```python
from build123d import *

# Parameters (mm, degrees)
F0_R     = 35
F1_DEPTH = 10


with BuildPart() as f1:
    # F0 (on Top) → F1 (new body)
    with BuildSketch(Plane.XY):
        Circle(F0_R)
    extrude(amount=F1_DEPTH)

    # F2 (on Front) → F3 (revolve)
    with BuildSketch(Plane.XZ):
        with BuildLine():
            Line((-26.283575, 70.897411), (-38.094532, 70.897411))
            Line((-38.094532, 70.897411), (-38.094532, 64.87011))
            Line((-38.094532, 64.87011), (-32.239489, 64.87011))
            Line((-32.239489, 64.87011), (-32.041561, 37.90903))
            ThreePointArc((-32.041561, 37.90903), (-31.961449, 35.927279), (-31.750564, 33.955151))
            Line((-31.750564, 33.955151), (-29.594322, 18.60863))
            ThreePointArc((-29.594322, 18.60863), (-26.252318, 12.453024), (-19.69159, 10))
            Line((-19.69159, 10), (-8.501253, 10))
            ThreePointArc((-8.501253, 10), (-9.799669, 10.171531), (-11.008998, 10.674353))
            Line((-11.008998, 10.674353), (-15.924307, 13.523948))
            ThreePointArc((-15.924307, 13.523948), (-19.204295, 16.590883), (-20.811549, 20.783871))
            Line((-20.811549, 20.783871), (-22.838106, 35.207384))
            ThreePointArc((-22.838106, 35.207384), (-22.985725, 36.587873), (-23.041804, 37.9751))
            Line((-23.041804, 37.9751), (-23.239732, 64.936179))
            Line((-23.239732, 64.936179), (-26.283575, 70.897411))
        make_face()
    revolve(axis=Axis((0, 0, 28.011288), (0, 0, 1)))


solid = f1.part
```
Part model, mm, in its own coordinate system. A direction names the side the tool comes from. Round coordinates to 2 decimals unless told otherwise and drop trailing zeros. Write each loop counter-clockwise with the first axis right and the second up, starting at its lowest first coordinate (ties: lowest second). Pieces come first, ordered by that corner, then holes.
Item 1: Cut at A-A, the plane z = 27. Give the cut face in (x, y), plus the area to 3 significant figures.
Results:
outline: circle Ø61.55 at (0, 0); hole circle Ø43.37 at (0, 0)
area: 1,500 mm2
Item 2: Which spindle directions (+Z, -Z, +X, -X, +Y, -Y) get a long thin tool onto all of the face, cutting with end or side? Do faces 1 (the cylindrical face through (-28, -21, 5)), 2 (the flat face through (31.22, -8.64, 64.87)), 3 (the conical face through (-11.498, -18.035, 24.891)). Say none if no direction does.
Results:
face 1: -Z
face 2: none
face 3: +Z
Item 3: Two-plate mould, pull along Y, no slides. Class faces 4 (the flat face through (0, 0, 10)), 5 (the conical face through (-13.93, 26.77, 22.76)), 6 (the conical face through (-22.073, -6.951, 51.644)), 7 (the flat face through (0, 0, 0)): +Y half, -Y half, draft (parallel to the pull), parting line (faces both ways), or undercut.
Results:
face 4: undercut
face 5: parting line
face 6: undercut
face 7: draft
Item 4: Drop flat-ended pins along their axis: pin 1 Ø21 at (x, y) = (15.5, -2) entering from +Z; pin 2 Ø23 at (x, y) = (-16, 0) entering from -Z; pin 3 Ø1 at (y, z) = (-12.5, 38.5) entering from +X; pin 4 Ø1 at (y, z) = (-19, 20.5) entering from +X. Give the stop position or say it passes through.
Results:
pin 1: stops at z = 70.59
pin 2: stops at z = 0
pin 3: stops at x = 29.71
pin 4: stops at x = 23.45
Item 5: Probe L1, parallel to Z at x = 32.5, y = -12; L2, parallel to X at y = 9, z = 61.5; L3, parallel to Y at x = 14.5, z = 60. List the from-to ranges inside material, lowest first.
Results:
L1: z = 0 to 10, 64.87 to 70.9
L2: x = -30.93 to -21.4, 21.4 to 30.93
L3: y = -28.75 to -18.11, 18.11 to 28.75
